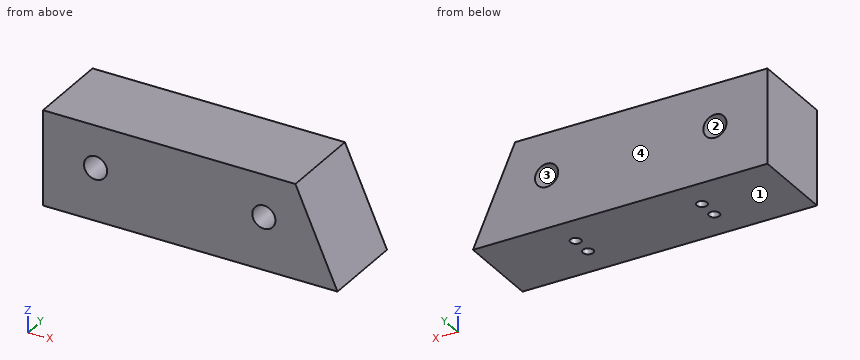
from build123d import *

# Parameters (mm, degrees)
SKETCH1_W           = 140
SKETCH1_H           = 40
BOSS_EXTRUDE1_DEPTH = 45
SKETCH2_R           = 5.5
CUT_EXTRUDE1_DEPTH  = 153.397506541
SKETCH3_R           = 2.5
CUT_EXTRUDE2_DEPTH  = 20


with BuildPart() as part:
    # Sketch1 → Boss-Extrude1 (new body)
    with BuildSketch(Plane.XY):
        with Locations((70, 20)):
            Rectangle(SKETCH1_W, SKETCH1_H)
    extrude(amount=BOSS_EXTRUDE1_DEPTH)

    # Sketch2 → Cut-Extrude1 (cut, through all)
    with BuildSketch(Plane.XZ):
        with Locations(Location((25, 25, 0), (0, 0, 270))):
            Circle(SKETCH2_R)
        with Locations(Location((105, 25, 0), (0, 0, 270))):
            Circle(SKETCH2_R)
        Polygon((120, 45), (140, 45), (140, 0), align=None)
    extrude(amount=-CUT_EXTRUDE1_DEPTH, mode=Mode.SUBTRACT)

    # Sketch3 → Cut-Extrude2 (cut)
    with BuildSketch(Plane(origin=(0, 0, 0), x_dir=(-1, 0, 0), z_dir=(0, 0, -1))):
        with Locations((-40, 25)):
            Circle(SKETCH3_R)
        with Locations((-100, 25)):
            Circle(SKETCH3_R)
        with Locations((-40, 15)):
            Circle(SKETCH3_R)
        with Locations((-100, 15)):
            Circle(SKETCH3_R)
    extrude(amount=-CUT_EXTRUDE2_DEPTH, mode=Mode.SUBTRACT)


solid = part.part
Part model, mm, in its own coordinate system. Face numbers are marked on the shaded views. Coordinates: 2 decimals unless noted, no trailing zeros. Loops run counter-clockwise (first coordinate to the right, second up) from the corner with the lowest first, then second, coordinate; pieces in that order, holes last. Notation, with made-up numbers: M 59,28.25 L 67,28.25 A11 cw 67,43.25 Z; hole C -35.5,29 d11. An arc over 180 degrees is marked long. Use a Markdown table: item, result. Add a question column.
Q1. Mould opens along Z. For the marked faces 1, 2, 3 and 4 say: +Z half, -Z half, draft (parallel to the pull), parting line (faces both ways), or undercut.
Q2. Cut at B-B (x = 105). Write the cut outline in (y, z).
Q3. Cut at C-C (y = 25). Write the cut outline in (x, z), and give its area (3 significant figures).
Q4. Pin check, flat tips, straight feed: P1, Ø1.5, axis at x = 101, y = 25.5, coming from the -Z side; P2, Ø1.5, axis at y = 18.5, z = 12.5, coming from the +X side; P3, Ø5, axis at y = 15, z = 40, coming from the +X side. Stop position of each tip, or through.
Q5. Cut at D-D (z = 15). Write the cut outline in (x, y), and give its area (3 significant figures).
Q6. Probe L1, parallel to Y at x = 100, z = 5.75; L2, parallel to X at y = 3.5, z = 25; L3, parallel to Y at x = 102, z = 2. List the from-to ranges inside material, lowest first.
Q7. Cut at A-A (z = 25.5). Write the cut outline in (x, y).
Worked out:
| question | item | result |
|---|---|---|
| 1 | face 1 | -Z half |
| 1 | face 2 | undercut |
| 1 | face 3 | undercut |
| 1 | face 4 | draft |
| 2 | outline | M 0,0 L 40,0 L 40,19.5 L 0,19.5 Z; M 0,30.5 L 40,30.5 L 40,45 L 0,45 Z |
| 3 | outline | M 0,0 L 37.5,0 L 37.5,20 L 42.5,20 L 42.5,0 L 97.5,0 L 97.5,20 L 102.5,20 L 102.5,0 L 140,0 L 120,45 L 0,45 Z; hole C 25,25 d11; hole C 105,25 d11 |
| 3 | area | 5,460 mm2 |
| 4 | P1 | stops at z = 20 |
| 4 | P2 | stops at x = 134.78 |
| 4 | P3 | stops at x = 123.33 |
| 5 | outline | M 0,0 L 133.33,0 L 133.33,40 L 0,40 Z; hole C 40,15 d5; hole C 40,25 d5; hole C 100,15 d5; hole C 100,25 d5 |
| 5 | area | 5,250 mm2 |
| 6 | L1 | y = 0 to 12.5, 17.5 to 22.5, 27.5 to 40 |
| 6 | L2 | x = 0 to 19.5, 30.5 to 99.5, 110.5 to 128.89 |
| 6 | L3 | y = 0 to 13.5, 16.5 to 23.5, 26.5 to 40 |
| 7 | outline | M 0,0 L 19.52,0 L 19.52,40 L 0,40 Z; M 30.48,0 L 99.52,0 L 99.52,40 L 30.48,40 Z; M 110.48,0 L 128.67,0 L 128.67,40 L 110.48,40 Z |
